The model under review builds one solid part; all positions refer to its coordinate system, in mm. A direction names the side the tool comes from. Give positions to 0.01 mm unless a question says otherwise; leave off trailing zeros. Order: outer loops, then holes, each group sorted by start corner. A loop starts at its lowest first (then second) coordinate and runs counter-clockwise, first axis right, second up. Notation, with made-up numbers: (30.5, 57.25) - (62.5, 57.25) arc R6 cw to (62.5, 62.25) - close; hole circle Ø2 at (58, 33.25). An arc over 180 degrees is marked (long way). Put each result on its own line as item: value.
```python
from build123d import *

# Parameters (mm, degrees)
SKETCH1_R           = 1.65
BOSS_EXTRUDE1_DEPTH = 3.8
CUT_EXTRUDE1_DEPTH  = 26.02878343
CIRPATTERN1_COUNT   = 12
SKETCH3_W           = 5.990659071
SKETCH3_H           = 5
BOSS_EXTRUDE2_DEPTH = 4
SKETCH4_R           = 2.5
CUT_EXTRUDE2_DEPTH  = 25.846159393


with BuildPart() as part:
    # Sketch1 → Boss-Extrude1 (new body)
    with BuildSketch(Plane.XY):
        with BuildLine():
            Line((-18, 2.5), (12.545643943, 2.5))
            ThreePointArc((12.545643943, 2.5), (24, 0), (12.545643943, -2.5))
            Line((12.545643943, -2.5), (-18, -2.5))
            ThreePointArc((-18, -2.5), (-20.5, 0), (-18, 2.5))
        make_face()
        with Locations(Location((-18, 0, 0), (0, 0, 180))):
            Circle(SKETCH1_R, mode=Mode.SUBTRACT)
    extrude(amount=BOSS_EXTRUDE1_DEPTH)

    # Sketch2 → Cut-Extrude1 (cut, through all)
    with BuildSketch(Plane.XY.offset(3.8)):
        with BuildLine():
            Line((20.008070513, 4.695554958), (19.882890915, 4.479152397))
            ThreePointArc((19.882890915, 4.479152397), (19.821496871, 4.016588638), (20.105, 3.64596695))
            ThreePointArc((20.105, 3.64596695), (20.567719361, 3.585756883), (20.937614306, 3.870207564))
            Line((20.937614306, 3.870207564), (21.062434622, 4.086817556))
            ThreePointArc((21.062434622, 4.086817556), (21.614093727, 4.455903836), (22.242640687, 4.242640687))
            ThreePointArc((22.242640687, 4.242640687), (21.131352886, 5.423662295), (19.552914271, 5.795554958))
            ThreePointArc((19.552914271, 5.795554958), (20.051879055, 5.357848898), (20.008070513, 4.695554958))
        make_face()
    cut_extrude1 = extrude(amount=-CUT_EXTRUDE1_DEPTH, mode=Mode.SUBTRACT)

    # CirPattern1: Cut-Extrude1 ×12 about axis
    cirpattern1_axis = Axis((18, 0, 0), (0, 0, 1))
    for i in range(1, CIRPATTERN1_COUNT):
        add(cut_extrude1.rotate(cirpattern1_axis, i * 360 / CIRPATTERN1_COUNT), mode=Mode.SUBTRACT)

    # Sketch3 → Boss-Extrude2 (add)
    with BuildSketch(Plane.XY.offset(3.8)):
        with Locations((13.282390893, 0)):
            Rectangle(SKETCH3_W, SKETCH3_H)
    extrude(amount=-BOSS_EXTRUDE2_DEPTH)

    # Sketch4 → Cut-Extrude2 (cut, through all)
    with BuildSketch(Plane.XY.offset(3.8)):
        with Locations((18, 0)):
            Circle(SKETCH4_R)
    extrude(amount=-CUT_EXTRUDE2_DEPTH, mode=Mode.SUBTRACT)


solid = part.part
```
(1) Wall thickness on L1, parallel to Y at x = -18, z = 1.25; L2, parallel to X at y = -0.5, z = 2.35; L3, parallel to X at y = 2, z = 3.55: over which ranges is each line inside the solid? List them lowest first.
The answers:
L1: -2.5 to -1.65, 1.65 to 2.5
L2: -20.45 to -19.57, -16.43 to 15.55, 20.45 to 22.47
L3: -19.5 to 16.5, 19.5 to 21.72, 22.68 to 23.46
(2) Take a section at A-A, the plane x = -17.5. Write out the cut boundary in (y, z).
The answers:
outline: (-2.5, 0) - (-1.57, 0) - (-1.57, 3.8) - (-2.5, 3.8) - close; (1.57, 0) - (2.5, 0) - (2.5, 3.8) - (1.57, 3.8) - close
(3) Clearance check with a flat-ended pin moving along its axis: pin 1 Ø5 at (x, y) = (19, 2.5) entering from -Z. State where the tip first meets the part, or that it passes through.
The answers:
pin 1: z = 0
(4) Take a section at B-B, the plane z = 1.8. Count the separate pieces of the cut face and the enclosed holes in it, then the cut area to 3 significant figures.
The answers:
separate pieces: 1
enclosed holes: 2
area: 221 mm^2
(5) The part is to be moulded in two halves that separate along Y. For faces 1 (the cylindrical face through (15.439, -3.584, 1.927)), 2 (the flat face through (21, 0, 0)), 3 (the cylindrical face through (15.5, 0.1, 1.8)), 4 (the cylindrical face through (-19.574, -0.496, 1.873)), say which applies: pulls with the +Y half, pulls with the -Y half, needs draft (parallel to the pull), parting line crosses it, or undercut.
The answers:
face 1: pulls with the -Y half
face 2: needs draft
face 3: undercut
face 4: undercut
(6) For faces 5 (the cylindrical face through (21.584, -2.561, 1.927)), 6 (the flat face through (-5, 0, 0)), 7 (the cylindrical face through (19.82, 4.02, 1.93)), list the 3-axis set-ups (+Z, -Z, +X, -X, +Y, -Y) from which the entire face can be reached by the end or side of a thin tool; tool diameter is ignored.
The answers:
face 5: +Z, -Z, +X
face 6: -Z, -X, +Y, -Y
face 7: +Z, -Z
